```python
from build123d import *

# Parameters (mm, degrees)
F1_DEPTH = 25.4
F2_T     = -3.9878
F3_DEPTH = 3.9878
F4_DEPTH = 3.9878


with BuildPart() as f1:
    # F0 (on Front) → F1 (new body)
    with BuildSketch(Plane.XZ):
        Polygon((0, -32.8910034207), (13.49375, -32.8910034207), (38.1, 39.1559594118), (0, 39.1559594118), (-38.1, 39.1559594118), (-13.49375, -32.8910034207), align=None)
    extrude(amount=F1_DEPTH)

    # F2
    f2_openings = [f1.faces().sort_by_distance(p)[0] for p in [
        (0, -25.4, 8.859288),
    ]]
    offset(amount=F2_T, openings=f2_openings)

    # F3 (cut, through all): a face of the model
    f3_faces = [f1.faces().sort_by_distance(p)[0] for p in [
        (0, -14.6939, -28.9032034207),
    ]]
    extrude(f3_faces, amount=-F3_DEPTH, mode=Mode.SUBTRACT)

    # F4 (cut, through all): a face of the model
    f4_faces = [f1.faces().sort_by_distance(p)[0] for p in [
        (0, -14.6939, 35.1681594118),
    ]]
    extrude(f4_faces, amount=-F4_DEPTH, mode=Mode.SUBTRACT)


solid = f1.part
```
Here's how the part is built. I have some questions about the finished solid (model axes, mm). A direction names the side the tool comes from. Coordinates: 2 decimals unless noted, no trailing zeros. Order: outer loops, then holes, each group sorted by start corner. A loop starts at its lowest first (then second) coordinate and runs counter-clockwise, first axis right, second up. Notation, with made-up numbers: (-0.5, 82) - (39.5, 82) arc R11 ccw to (39.5, 87) - close; hole circle Ø3 at (0, 43). An arc over 180 degrees is marked (long way). One line per question, with ' | ' between items. Start each with the question number.
1. If we section it at C-C (x = -14.5): Write out the boundary of the cut face in (y, z), and give its area (3 significant figures).
2. If we section it at D-D (z = 12): Write out the boundary of the cut face in (x, y), and give its area (3 significant figures).
3. I'm going to push flat-ended pins straight in: pin 1 Ø3 at (y, z) = (-10, -30.5) entering from -X; pin 2 Ø1 at (x, z) = (23.5, 21.5) entering from -Y; pin 3 Ø1 at (y, z) = (-11, 10) entering from +X. Where does each tip first touch, or does it pass through?
4. If we mould it in two halves opening along X, with no side actions, what happens to faces 1 (the flat face through (-21.736, -14.544, 3.581)), 2 (the flat face through (24, -25.4, 3)), 3 (the flat face through (25.625, -12.522, 2.628))? For each: released by +X, released by -X, zero draft, split by the parting line, or undercut.
5. If we section it at A-A (y = -23.25): Write out the boundary of the cut face in (x, z).
6. If we section it at B-B (z = -18): Write out the boundary of the cut face in (x, y), and give its area (3 significant figures).
7. Which directions (+Z, -Z, +X, -X, +Y, -Y) give clear straight access to the entire face, cutting with the end or side of a thin tool? Please do faces 4 (the flat face through (-32.524, -15, 37)), 5 (the flat face through (-24, -25.4, 6)), 6 (the flat face through (10.642, -15, -31)).
8. Please list where these lines run through material, in increasing order: line 1 along Y through (x, z) = (17, -1.5); line 2 along X through (y, z) = (-10.25, 23); line 3 along X through (y, z) = (-15.25, 16.5). Write a range as [from, to].
Model answer:
1) outline: (-25.4, -29.94) - (0, -29.94) - (0, 39.16) - (-3.99, 39.16) - (-3.99, -17.61) - (-25.4, -17.61) - close | area: 540 mm²
2) outline: (-28.83, -25.4) - (-24.61, -25.4) - (-24.61, -3.99) - (24.61, -3.99) - (24.61, -25.4) - (28.83, -25.4) - (28.83, 0) - (-28.83, 0) - close | area: 410 mm²
3) pin 1: stops at x = -14.82 | pin 2: stops at y = -3.99 | pin 3: stops at x = 28.31
4) face 1: undercut | face 2: zero draft | face 3: released by +X
5) outline: (-38.1, 39.16) - (-13.49, -32.89) - (-10.64, -32.89) - (-10.64, -28.9) - (-32.52, 35.17) - (-32.52, 39.16) - close; (10.64, -32.89) - (13.49, -32.89) - (38.1, 39.16) - (32.52, 39.16) - (32.52, 35.17) - (10.64, -28.9) - close
6) outline: (-18.58, -25.4) - (-14.37, -25.4) - (-14.37, -3.99) - (14.37, -3.99) - (14.37, -25.4) - (18.58, -25.4) - (18.58, 0) - (-18.58, 0) - close | area: 329 mm²
7) face 4: +Z, -Y | face 5: +Z, -Z, +X, -X, -Y | face 6: +Z, -Z, -Y
8) line 1: y = [-3.99, 0] | line 2: x = [-32.58, -28.37], [28.37, 32.58] | line 3: x = [-30.36, -26.15], [26.15, 30.36]
